Read the model definition and answer for the solid it produces. Units are mm, in the model's axes. Face numbers are marked on the shaded views. A direction names the side the tool comes from. Round coordinates to 2 decimals unless told otherwise and drop trailing zeros. Order: outer loops, then holes, each group sorted by start corner. A loop starts at its lowest first (then second) coordinate and runs counter-clockwise, first axis right, second up. Notation, with made-up numbers: (22.25, 49.25) - (31.25, 49.25) arc R17 cw to (31.25, 70.25) - close; hole circle Ø7 at (83.25, 62.25). An arc over 180 degrees is marked (long way). One line per question, with ' | ' between items. Start each with the question number.
1) Flat-ended cylindrical pins translate along their axes: pin 1 (2 mm diameter, centred on x = 8.5, z = -5.5, fed in from +Y); pin 2 (4 mm diameter, centred on x = 6.5, y = -6.5, fed in from +Z); pin 3 (2 mm diameter, centred on x = -1, y = -1, fed in from +Z). Find the tip coordinate at first contact, or state that the pin passes through.
2) The part is cut by section C-C, the plane z = -2.25. Give the vertices of the cut face in (x, y), plus the area to 3 significant figures.
3) The part is cut by section A-A, the plane z = 6.5. Count the separate pieces of the cut face and the enclosed holes in it, plus the area to 3 significant figures.
4) The mould has two halves that part along X. Classify the marked faces 1, 2 and 3: pulls with the +X half, pulls with the -X half, needs draft (parallel to the pull), parting line crosses it, or undercut.
5) The part is cut by section B-B, the plane x = -22.5. Give the vertices of the cut face in (y, z).
6) Straight lines are drawn through the part: line 1 (Y direction, x = 0, z = 8.3); line 2 (Y direction, x = 0, z = -11.5); line 3 (Z direction, x = 23, y = -9). For each, find the intervals that lie inside material, in ascending order. Write a range as from..to.
7) For the marked faces 4, 5, 6 and 7, determine the directions among +Z, -Z, +X, -X, +Y, -Y from which every point of the face is accessible in a straight line to the end or side of a thin tool.
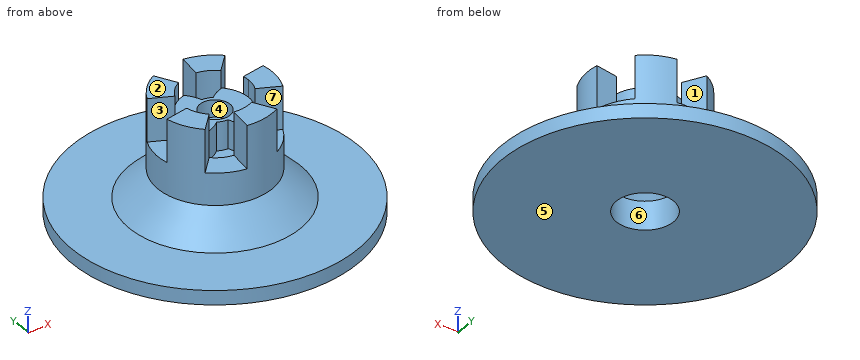
from build123d import *

# Parameters (mm, degrees)
SKETCH11_R          = 3.3672
CUT_EXTRUDE5_DEPTH  = 3.81
SKETCH11_5_R        = 3.3672
CUT_EXTRUDE7_DEPTH  = 7.62
CUT_EXTRUDE8_DEPTH  = 10.16
SKETCH13_R          = 6.35
CUT_EXTRUDE10_DEPTH = 12.192
CHAMFER1_SIZE       = 5.842
CHAMFER2_SIZE       = 6.35
CUT_EXTRUDE11_DEPTH = 9.525


with BuildPart() as part:
    # Sketch2 → Revolve1 (revolve)
    with BuildSketch(Plane(origin=(0, 0, 0), x_dir=(0, 0, -1), z_dir=(1, 0, 0))):
        Polygon((-13.081, 0), (-13.081, 9.525), (-13.081, 12.7), (-9.906, 12.7), (9.906, 12.7), (9.906, 31.75), (13.081, 31.75), (13.081, 0), align=None)
    revolve(axis=Axis((0, 0, -13.081), (0, 0, 1)))

    # Sketch11 → Cut-Extrude5 (cut)
    # profile 1 of 4: a face of its own
    with BuildSketch(Plane.XY.offset(13.081)):
        with BuildLine():
            ThreePointArc((-5.295442149, -5.31114794), (-1.969377828, -7.23681912), (1.873833325, -7.262144908))
            ThreePointArc((1.873833325, -7.262144908), (0.767613275, -5.832118974), (0.033615166, -4.179864833))
            ThreePointArc((0.033615166, -4.179864833), (-1.097599909, -4.033320523), (-2.147079662, -3.586425647))
            ThreePointArc((-2.147079662, -3.586425647), (-3.617120551, -4.638887883), (-5.295442149, -5.31114794))
        make_face()
    # profile 2 of 4: a face of its own
    with BuildSketch(Plane.XY.offset(13.081)):
        with BuildLine():
            ThreePointArc((7.5, 0), (6.926969616, 2.875255109), (5.295442149, 5.31114794))
            ThreePointArc((5.295442149, 5.31114794), (3.617120551, 4.638887883), (2.147079662, 3.586425647))
            ThreePointArc((2.147079662, 3.586425647), (1.097599909, 4.033320523), (-0.033615166, 4.179864833))
            ThreePointArc((-0.033615166, 4.179864833), (-0.767613275, 5.832118974), (-1.873833325, 7.262144908))
            ThreePointArc((-1.873833325, 7.262144908), (-7.23681912, 1.969377828), (-5.295442149, -5.31114794))
            ThreePointArc((-5.295442149, -5.31114794), (-3.617120551, -4.638887883), (-2.147079662, -3.586425647))
            ThreePointArc((-2.147079662, -3.586425647), (-1.097599909, -4.033320523), (0.033615166, -4.179864833))
            ThreePointArc((0.033615166, -4.179864833), (0.767613275, -5.832118974), (1.873833325, -7.262144908))
            ThreePointArc((1.873833325, -7.262144908), (5.928901666, -4.593269536), (7.5, 0))
        make_face()
        Circle(SKETCH11_R, mode=Mode.SUBTRACT)
    # profile 3 of 4: a face of its own
    with BuildSketch(Plane.XY.offset(13.081)):
        Circle(SKETCH11_R)
    # profile 4 of 4: a face of its own
    with BuildSketch(Plane.XY.offset(13.081)):
        with BuildLine():
            ThreePointArc((2.147079662, 3.586425647), (3.617120551, 4.638887883), (5.295442149, 5.31114794))
            ThreePointArc((5.295442149, 5.31114794), (1.969377828, 7.23681912), (-1.873833325, 7.262144908))
            ThreePointArc((-1.873833325, 7.262144908), (-0.767613275, 5.832118974), (-0.033615166, 4.179864833))
            ThreePointArc((-0.033615166, 4.179864833), (1.097599909, 4.033320523), (2.147079662, 3.586425647))
        make_face()
    extrude(amount=-CUT_EXTRUDE5_DEPTH, mode=Mode.SUBTRACT)

    # Sketch11<5> → Cut-Extrude7 (cut)
    with BuildSketch(Plane.XY.offset(13.081)):
        Circle(SKETCH11_5_R)
    extrude(amount=-CUT_EXTRUDE7_DEPTH, mode=Mode.SUBTRACT)

    # Sketch11<6> → Cut-Extrude8 (cut)
    with BuildSketch(Plane.XY.offset(13.081)):
        with BuildLine():
            ThreePointArc((-5.295442149, -5.31114794), (-1.969377828, -7.23681912), (1.873833325, -7.262144908))
            ThreePointArc((1.873833325, -7.262144908), (0.767613275, -5.832118974), (0.033615166, -4.179864833))
            ThreePointArc((0.033615166, -4.179864833), (-1.097599909, -4.033320523), (-2.147079662, -3.586425647))
            ThreePointArc((-2.147079662, -3.586425647), (-3.617120551, -4.638887883), (-5.295442149, -5.31114794))
        make_face()
        with BuildLine():
            ThreePointArc((2.147079662, 3.586425647), (3.617120551, 4.638887883), (5.295442149, 5.31114794))
            ThreePointArc((5.295442149, 5.31114794), (1.969377828, 7.23681912), (-1.873833325, 7.262144908))
            ThreePointArc((-1.873833325, 7.262144908), (-0.767613275, 5.832118974), (-0.033615166, 4.179864833))
            ThreePointArc((-0.033615166, 4.179864833), (1.097599909, 4.033320523), (2.147079662, 3.586425647))
        make_face()
    extrude(amount=-CUT_EXTRUDE8_DEPTH, mode=Mode.SUBTRACT)

    # Sketch13 → Cut-Extrude10 (cut)
    with BuildSketch(Plane(origin=(0, 0, -13.081), x_dir=(-1, 0, 0), z_dir=(0, 0, -1))):
        Circle(SKETCH13_R)
    extrude(amount=-CUT_EXTRUDE10_DEPTH, mode=Mode.SUBTRACT)

    # Chamfer1
    chamfer1_edges = [part.edges().sort_by_distance(p)[0] for p in [
        (6.35, 0, -0.889),
    ]]
    chamfer(chamfer1_edges, length=CHAMFER1_SIZE)

    # Chamfer2
    chamfer2_edges = [part.edges().sort_by_distance(p)[0] for p in [
        (0, -12.7, -9.906),
    ]]
    chamfer(chamfer2_edges, length=CHAMFER2_SIZE)

    # Sketch14 → Cut-Extrude11 (cut)
    with BuildSketch(Plane.XY.offset(13.081)):
        with BuildLine():
            Line((-6.77593781, 3.215068708), (-11.473921358, 5.444183013))
            ThreePointArc((-11.473921358, 5.444183013), (-12.594692746, 1.632089038), (-12.482607856, -2.339765182))
            Line((-12.482607856, -2.339765182), (-7.371618813, -1.381751092))
            ThreePointArc((-7.371618813, -1.381751092), (-7.437810677, 0.963832109), (-6.77593781, 3.215068708))
        make_face()
        with BuildLine():
            ThreePointArc((1.632089038, 12.594692746), (-2.339765182, 12.482607856), (-6.082586885, 11.148638338))
            Line((-6.082586885, 11.148638338), (-3.592078869, 6.583841538))
            ThreePointArc((-3.592078869, 6.583841538), (-1.381751092, 7.371618813), (0.963832109, 7.437810677))
            Line((0.963832109, 7.437810677), (1.632089038, 12.594692746))
        make_face()
        with BuildLine():
            ThreePointArc((12.482607856, 2.339765182), (11.148638338, 6.082586885), (8.723362422, 9.230002603))
            Line((8.723362422, 9.230002603), (5.151591981, 5.450788939))
            ThreePointArc((5.151591981, 5.450788939), (6.583841538, 3.592078869), (7.371618813, 1.381751092))
            Line((7.371618813, 1.381751092), (12.482607856, 2.339765182))
        make_face()
        with BuildLine():
            Line((3.592078869, -6.583841538), (6.082586885, -11.148638338))
            ThreePointArc((6.082586885, -11.148638338), (9.230002603, -8.723362422), (11.473921358, -5.444183013))
            Line((11.473921358, -5.444183013), (6.77593781, -3.215068708))
            ThreePointArc((6.77593781, -3.215068708), (5.450788939, -5.151591981), (3.592078869, -6.583841538))
        make_face()
        with BuildLine():
            Line((-5.151591981, -5.450788939), (-8.723362422, -9.230002603))
            ThreePointArc((-8.723362422, -9.230002603), (-5.444183013, -11.473921358), (-1.632089038, -12.594692746))
            Line((-1.632089038, -12.594692746), (-0.963832109, -7.437810677))
            ThreePointArc((-0.963832109, -7.437810677), (-3.215068708, -6.77593781), (-5.151591981, -5.450788939))
        make_face()
    extrude(amount=-CUT_EXTRUDE11_DEPTH, mode=Mode.SUBTRACT)


solid = part.part
Values:
1) pin 1: stops at y = 13.29 | pin 2: stops at z = 9.27 | pin 3: stops at z = 5.46
2) outline: circle Ø25.4 at (0, 0); hole circle Ø3.74 at (0, 0) | area: 496 mm^2
3) separate pieces: 2 | enclosed holes: 1 | area: 275 mm^2
4) face 1: undercut | face 2: needs draft | face 3: pulls with the -X half
5) outline: (-22.4, -13.08) - (22.4, -13.08) - (22.4, -9.91) - (-22.4, -9.91) - close
6) line 1: y = -12.7..-7.5, -4.18..-3.37, 3.37..4.18 | line 2: y = -31.75..-6.35, 6.35..31.75 | line 3: z = -13.08..-9.91
7) face 4: +Z | face 5: -Z, +X, -X, +Y, -Y | face 6: -Z | face 7: +Z, -Y
